from build123d import *

# Parameters (mm, degrees)
F2_R     = 25.921407
F3_DEPTH = 25


with BuildPart() as f1:
    # F0 (on Front) → F1 (revolve)
    with BuildSketch(Plane.XZ):
        Polygon((0, 10.126797), (0, 0), (31.009387, 0), (31.009387, 10.126797), (39.983399, 10.126797), (39.983399, 34.21212), (34.762897, 34.21212), (34.762897, 19.85573), (23.669325, 10.126797), align=None)
    revolve(axis=Axis((0, 0, 5.063399), (0, 0, -1)))

    # F2 (on Top) → F3 (cut)
    with BuildSketch(Plane.XY):
        Circle(F2_R)
    extrude(amount=F3_DEPTH, mode=Mode.SUBTRACT)


solid = f1.part
Geometry: final body of the model. Coordinates: model frame, mm. A direction names the side the tool comes from. Coordinates: 2 decimals unless noted, no trailing zeros. Order: outer loops, then holes, each group sorted by start corner. A loop starts at its lowest first (then second) coordinate and runs counter-clockwise, first axis right, second up. Notation, with made-up numbers: (-5, 75.25) - (51, 75.25) arc R6 ccw to (51, 81.25) - close; hole circle Ø8 at (69.25, 32.5). An arc over 180 degrees is marked (long way). Use one line per item in the form item = value.
1) Section C-C (z = 3.5). Return loops of the section in (x, y).
Solutions:
outline = circle Ø62.02 at (0, 0); hole circle Ø51.84 at (0, 0)
2) Mould query, pull axis X, two halves, no side actions, for faces 1 (the face through (24.724, 7.786, 5.966)), 2 (the face through (7.04, 25.12, 0)), 3 (the face through (-8.668, 39.033, 22.338)). Classes: +X half, -X half, draft (parallel to the pull), parting line (faces both ways), or undercut.
Solutions:
face_1 = undercut
face_2 = draft
face_3 = parting line
3) Section A-A (y = 0). Return loops of the section in (x, z).
Solutions:
outline = (-39.98, 10.13) - (-31.01, 10.13) - (-31.01, 0) - (-25.92, 0) - (-25.92, 12.1) - (-34.76, 19.86) - (-34.76, 34.21) - (-39.98, 34.21) - close; (25.92, 0) - (31.01, 0) - (31.01, 10.13) - (39.98, 10.13) - (39.98, 34.21) - (34.76, 34.21) - (34.76, 19.86) - (25.92, 12.1) - close
4) Set-up query: faces 4 (the face through (-12, -33, 34.212)), 5 (the face through (-21, 24, 10.127)), 6 (the face through (33.16, -10.44, 26.93)). Return all of +Z, -Z, +X, -X, +Y, -Y with unobstructed straight access to the full face (end or side cutting, diameter ignored); none if empty.
Solutions:
face_4 = +Z, +X, -X, +Y, -Y
face_5 = -Z
face_6 = +Z
5) Pin query (flat end, axial travel): pin 1 (12 mm diameter, centred on x = -19, z = 9.5, fed in from -Y); pin 2 (3 mm diameter, centred on y = 29.5, z = 10, fed in from +X); pin 3 (3 mm diameter, centred on x = 1.5, z = 23, fed in from -Y). Return the tip coordinate at first contact, or that it passes through.
Solutions:
pin_1 = -37.8
pin_2 = 28.54
pin_3 = -39.98
6) Ray query, L1, parallel to X at y = 0, z = 27; L2, parallel to Y at x = 0, z = 6. Return the intervals inside material, ascending.
Solutions:
L1 = -39.98 to -34.76, 34.76 to 39.98
L2 = -31.01 to -25.92, 25.92 to 31.01
